Read the model definition and answer for the solid it produces. Units are mm, in the model's axes. A direction names the side the tool comes from. Give positions to 0.01 mm unless a question says otherwise; leave off trailing zeros. Order: outer loops, then holes, each group sorted by start corner. A loop starts at its lowest first (then second) coordinate and runs counter-clockwise, first axis right, second up. Notation, with made-up numbers: (-21, 16.5) -> (-15, 16.5) arc R12 cw to (-15, 37.5) -> close; hole circle Ø7 at (-15.75, 85.5). An arc over 180 degrees is marked (long way). Use one line per item in the form item = value.
```python
from build123d import *

# Parameters (mm, degrees)
SKETCH_R     = 50.8
PAD_DEPTH    = 152.4
SKETCH001_R  = 9.652
POCKET_DEPTH = 79.402154


with BuildPart() as part:
    # Sketch → Pad (new body)
    with BuildSketch(Plane(origin=(0, 0, -76.2), x_dir=(1, 0, 0), z_dir=(0, 0, -1))):
        with BuildLine():
            ThreePointArc((62.205505, -6.599598), (62.554612, 0), (62.205505, 6.599598))
            Line((62.205505, 6.599598), (108.01374, 6.599598))
            Line((108.01374, 6.599598), (108.01374, 16.846542))
            Line((108.01374, 16.846542), (60.243452, 16.846542))
            ThreePointArc((60.243452, 16.846542), (0, 62.554612), (-60.243452, 16.846542))
            Line((-108.01374, 16.846542), (-60.243452, 16.846542))
            Line((-108.01374, 6.599598), (-108.01374, 16.846542))
            Line((-62.205505, 6.599598), (-108.01374, 6.599598))
            ThreePointArc((-62.205505, 6.599598), (-62.554612, 0), (-62.205505, -6.599598))
            Line((-62.205505, -6.599598), (-108.01374, -6.599598))
            Line((-108.01374, -6.599598), (-108.01374, -16.846542))
            Line((-108.01374, -16.846542), (-60.243452, -16.846542))
            ThreePointArc((-60.243452, -16.846542), (0, -62.554612), (60.243452, -16.846542))
            Line((108.01374, -16.846542), (60.243452, -16.846542))
            Line((108.01374, -6.599598), (108.01374, -16.846542))
            Line((62.205505, -6.599598), (108.01374, -6.599598))
        make_face()
        Circle(SKETCH_R, mode=Mode.SUBTRACT)
    extrude(amount=PAD_DEPTH)

    # Sketch001 → Pocket (cut, through all)
    with BuildSketch(Plane(origin=(0, -16.846542, -76.2), x_dir=(-1, 0, 0), z_dir=(0, -1, 0))):
        with Locations((-84.128596, 76.2)):
            Circle(SKETCH001_R)
        with Locations((84.128596, 76.2)):
            Circle(SKETCH001_R)
    extrude(amount=-POCKET_DEPTH, mode=Mode.SUBTRACT)


solid = part.part
```
Item 1: The part is cut by section D-D on z = -194.5. Give the vertices of the cut face in (x, y).
Checks:
outline = (-108.01, -16.85) -> (-60.24, -16.85) arc R62.55 ccw to (60.24, -16.85) -> (108.01, -16.85) -> (108.01, -6.6) -> (62.21, -6.6) arc R62.55 ccw to (62.21, 6.6) -> (108.01, 6.6) -> (108.01, 16.85) -> (60.24, 16.85) arc R62.55 ccw to (-60.24, 16.85) -> (-108.01, 16.85) -> (-108.01, 6.6) -> (-62.21, 6.6) arc R62.55 ccw to (-62.21, -6.6) -> (-108.01, -6.6) -> close; hole circle Ø101.6 at (0, 0)
Item 2: Which of the six approach directions +Z, -Z, +X, -X, +Y, -Y give full straight-line access (tool end or side, diameter ignored) to faces 1 (the flat face through (95, 16.847, -151)), 2 (the flat face through (-95, 6.6, -151)), 3 (the flat face through (-95, -16.847, -151)), 4 (the flat face through (95, -16.847, -151)), 5 (the flat face through (95, -6.6, -151))?
Checks:
face_1 = +Z, -Z, +X, +Y
face_2 = +Z, -Z, -X
face_3 = +Z, -Z, -X, -Y
face_4 = +Z, -Z, +X, -Y
face_5 = +Z, -Z, +X
Item 3: The part is cut by section A-A on z = -152.4. State how many separate pieces and enclosed holes the cut face has, and give its area (3 significant figures).
Checks:
separate_pieces = 5
enclosed_holes = 1
area = 5,310 mm²
Item 4: Determine the mould class of faces 6 (the flat face through (-1, -51, -228.6)), 7 (the flat face through (-1, -51, -76.2)), 8 (the cylindrical face through (-74.486, 11.651, -152.824)), 9 (the cylindrical face through (1.137, -62.544, -151.333)) for opening direction Z: +Z half, -Z half, draft (parallel to the pull), parting line (faces both ways), or undercut.
Checks:
face_6 = -Z half
face_7 = +Z half
face_8 = undercut
face_9 = draft
Item 5: Straight lines are drawn through the part: L1, parallel to Y at x = 63, z = -168; L2, parallel to X at y = -13.5, z = -152.4; L3, parallel to X at y = 13, z = -152.4. For each, find the intervals that lie inside material, in ascending order. Write a range as from..to.
Checks:
L1 = -16.85..-6.6, 6.6..16.85
L2 = -108.01..-93.78, -74.48..-48.97, 48.97..74.48, 93.78..108.01
L3 = -108.01..-93.78, -74.48..-49.11, 49.11..74.48, 93.78..108.01
Item 6: The part is cut by section B-B on x = 0. Give the vertices of the cut face in (y, z), and give its area (3 significant figures).
Checks:
outline = (-62.55, -228.6) -> (-50.8, -228.6) -> (-50.8, -76.2) -> (-62.55, -76.2) -> close; (50.8, -228.6) -> (62.55, -228.6) -> (62.55, -76.2) -> (50.8, -76.2) -> close
area = 3,580 mm²
Item 7: Given pin 1 Ø1.5 at (y, z) = (-35, -203) entering from -X; pin 2 Ø5 at (y, z) = (-30, -192.5) entering from -X; pin 3 Ø13.5 at (x, z) = (-74, -123) entering from -Y; pin 4 Ø15.5 at (x, z) = (-84.13, -152.4) entering from -Y, each flat-ended and moving along its own axis, determine where each tip first touches the part or whether it passes through.
Checks:
pin_1 = -52.35
pin_2 = -56.19
pin_3 = -16.85
pin_4 = through
